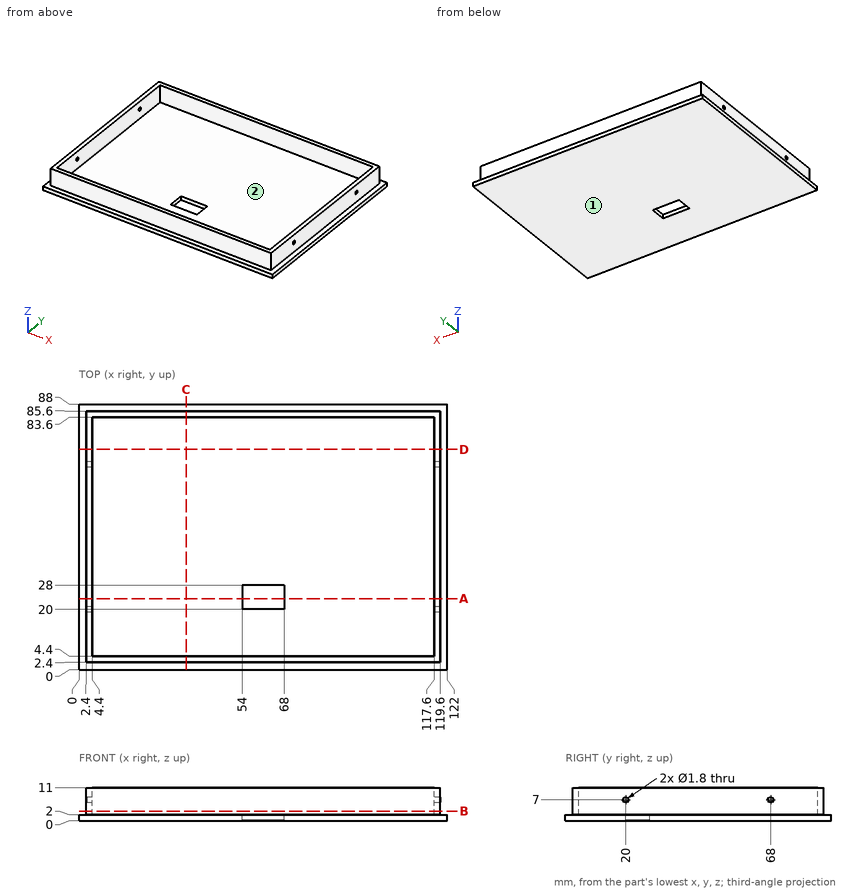
The figure shows three views and two pictorial views of one solid part (mm, origin at its lowest corner). Answer the questions. Round coordinates to 2 decimals unless told otherwise and drop trailing zeros. Write each loop counter-clockwise with the first axis right and the second up, starting at its lowest first coordinate (ties: lowest second). Pieces come first, ordered by that corner, then holes. Notation, with made-up numbers: (89, -37) -> (94, -37) arc R11 ccw to (94, -27) -> close; hole circle Ø4 at (-27, 40). An arc over 180 degrees is marked (long way). Answer as a JSON object with one key per item and string values. Group by question number.
Q1. Section A-A (y = 23.5) is taken. Write down the section's boundary in (x, z), plus the area to 3 significant figures.
Q2. Section D-D (y = 73) is taken. Write down the section's boundary in (x, z).
Q3. Each of these flat-tipped pins is pushed along its axis until it touches: pin 1 Ø6 at (y, z) = (67, 9.5) entering from -X; pin 2 Ø2.5 at (y, z) = (68, 7) entering from +X; pin 3 Ø2.5 at (x, z) = (55, 5) entering from +Y. Where does it stop, or does it pass through?
Q4. Section B-B (z = 3.25) is taken. Write down the section's boundary in (x, y), plus the area to 3 significant figures.
Q5. Straight lines are drawn through the part: line 1 along Y through (x, z) = (3.75, 7); line 2 along Z through (x, y) = (118, 20); line 3 along Y through (x, z) = (20, 10.5). For each, find the intervals that lie inside material, in ascending order.
Q6. Section C-C (x = 35.5) is taken. Write down the section's boundary in (y, z).
Q7. Determine the mould class of the marked faces 1 and 2 for opening direction X: pulls with the +X half, pulls with the -X half, needs draft (parallel to the pull), parting line crosses it, or undercut.
Check values:
{
 "1": {"outline": "(0, 0) -> (54, 0) -> (54, 2) -> (4.4, 2) -> (4.4, 11) -> (2.4, 11) -> (2.4, 2) -> (0, 2) -> close; (68, 0) -> (122, 0) -> (122, 2) -> (119.6, 2) -> (119.6, 11) -> (117.6, 11) -> (117.6, 2) -> (68, 2) -> close", "area": "252 mm^2"},
 "2": {"outline": "(0, 0) -> (122, 0) -> (122, 2) -> (119.6, 2) -> (119.6, 11) -> (117.6, 11) -> (117.6, 2) -> (4.4, 2) -> (4.4, 11) -> (2.4, 11) -> (2.4, 2) -> (0, 2) -> close"},
 "3": {"pin 1": "x = 2.4", "pin 2": "x = 119.6", "pin 3": "y = 85.6"},
 "4": {"outline": "(2.4, 2.4) -> (119.6, 2.4) -> (119.6, 85.6) -> (2.4, 85.6) -> close; hole (4.4, 4.4) -> (117.6, 4.4) -> (117.6, 83.6) -> (4.4, 83.6) -> close", "area": "786 mm^2"},
 "5": {"line 1": "2.4 to 19.1, 20.9 to 67.1, 68.9 to 85.6", "line 2": "0 to 6.1, 7.9 to 11", "line 3": "2.4 to 4.4, 83.6 to 85.6"},
 "6": {"outline": "(0, 0) -> (88, 0) -> (88, 2) -> (85.6, 2) -> (85.6, 11) -> (83.6, 11) -> (83.6, 2) -> (4.4, 2) -> (4.4, 11) -> (2.4, 11) -> (2.4, 2) -> (0, 2) -> close"},
 "7": {"face 1": "needs draft", "face 2": "undercut"}
}
